```python
from build123d import *

# Parameters (mm, degrees)
SKETCH1_W           = 495.5921
SKETCH1_H           = 147.69846
BOSS_EXTRUDE1_DEPTH = 3.175
SKETCH2_W           = 76.2
SKETCH2_H           = 3.175
BOSS_EXTRUDE2_DEPTH = 6.35
SKETCH3_W           = 3.175
SKETCH3_H           = 188.73216
CUT_EXTRUDE1_DEPTH  = 3.175
SKETCH4_W           = 3.175
SKETCH4_H           = 94.36608
BOSS_EXTRUDE3_DEPTH = 3.175
SKETCH5_W           = 96.57842
SKETCH5_H           = 18.04416
BOSS_EXTRUDE4_DEPTH = 3.175
SKETCH6_W           = 96.577155917
SKETCH6_H           = 2.032
CUT_EXTRUDE2_DEPTH  = 523.024547982
SKETCH7_W           = 6.603370135
SKETCH7_H           = 28.867559882
CUT_EXTRUDE3_DEPTH  = 523.024547982


with BuildPart() as part:
    # Sketch1 → Boss-Extrude1 (new body)
    with BuildSketch(Plane(origin=(0, 0, 0), x_dir=(1, 0, 0), z_dir=(0, 1, 0))):
        with Locations((247.79605, 73.84923)):
            Rectangle(SKETCH1_W, SKETCH1_H)
    extrude(amount=BOSS_EXTRUDE1_DEPTH)

    # Sketch2 → Boss-Extrude2 (add)
    with BuildSketch(Plane(origin=(0, 0, -147.69846), x_dir=(-1, 0, 0), z_dir=(0, 0, -1))):
        with Locations((-447.30289, 1.5875)):
            Rectangle(SKETCH2_W, SKETCH2_H)
        with Locations((-347.54947, 1.5875)):
            Rectangle(SKETCH2_W, SKETCH2_H)
        with Locations((-247.79605, 1.5875)):
            Rectangle(SKETCH2_W, SKETCH2_H)
        with Locations((-148.04263, 1.5875)):
            Rectangle(SKETCH2_W, SKETCH2_H)
        with Locations((-47.895498166, 1.5875)):
            Rectangle(SKETCH2_W, SKETCH2_H)
    extrude(amount=BOSS_EXTRUDE2_DEPTH)

    # Sketch3 → Cut-Extrude1 (cut)
    with BuildSketch(Plane(origin=(0, 3.175, 0), x_dir=(1, 0, 0), z_dir=(0, 1, 0))):
        with Locations((397.42618, 0)):
            Rectangle(SKETCH3_W, SKETCH3_H)
        with Locations((297.67276, 0)):
            Rectangle(SKETCH3_W, SKETCH3_H)
        with Locations((197.91934, 0)):
            Rectangle(SKETCH3_W, SKETCH3_H)
        with Locations((98.167184083, 0)):
            Rectangle(SKETCH3_W, SKETCH3_H)
    extrude(amount=-CUT_EXTRUDE1_DEPTH, mode=Mode.SUBTRACT)

    # Sketch4 → Boss-Extrude3 (add, through all)
    with BuildSketch(Plane(origin=(0, 3.175, 0), x_dir=(1, 0, 0), z_dir=(0, 1, 0))):
        with Locations((-1.5875, 100.51542)):
            Rectangle(SKETCH4_W, SKETCH4_H)
        with Locations((497.1796, 100.51542)):
            Rectangle(SKETCH4_W, SKETCH4_H)
    extrude(amount=-BOSS_EXTRUDE3_DEPTH)

    # Sketch5 → Boss-Extrude4 (add, through all)
    with BuildSketch(Plane(origin=(0, 3.175, 0), x_dir=(1, 0, 0), z_dir=(0, 1, 0))):
        with Locations((247.79605, -9.02208)):
            Rectangle(SKETCH5_W, SKETCH5_H)
        with Locations((347.54947, -9.02208)):
            Rectangle(SKETCH5_W, SKETCH5_H)
        Polygon((429.9839, -18.04416), (431.560448611, -18.04416), (431.560448611, 0), (423.633900075, 0), (399.210535917, 0), (399.210535917, -18.04416), align=None)
        Polygon((495.5921, 0), (484.468648611, -18.04416), (459.500448611, -18.04416), (459.500448611, 0), (484.468648611, 0), align=None)
        Polygon((0, 0), (10.417800633, -18.04416), (96.579684083, -18.04416), (96.579684083, 0), align=None)
    extrude(amount=-BOSS_EXTRUDE4_DEPTH)

    # Sketch6 → Cut-Extrude2 (cut, through all)
    with BuildSketch(Plane(origin=(0, 3.175, 0), x_dir=(1, 0, 0), z_dir=(0, 1, 0))):
        with Locations((148.043262041, 1.016)):
            Rectangle(SKETCH6_W, SKETCH6_H)
    extrude(amount=-CUT_EXTRUDE2_DEPTH, mode=Mode.SUBTRACT)

    # Sketch7 → Cut-Extrude3 (cut, through all)
    with BuildSketch(Plane(origin=(0, 3.175, 0), x_dir=(1, 0, 0), z_dir=(0, 1, 0))):
        with Locations((94.765629101, -7.077939941)):
            Rectangle(SKETCH7_W, SKETCH7_H)
    extrude(amount=-CUT_EXTRUDE3_DEPTH, mode=Mode.SUBTRACT)


solid = part.part
```
The listing builds one solid part. Answer for the finished solid, in the listing's coordinates (mm). Give positions to 0.01 mm unless a question says otherwise; leave off trailing zeros. Order: outer loops, then holes, each group sorted by start corner. A loop starts at its lowest first (then second) coordinate and runs counter-clockwise, first axis right, second up.
Item 1: Find the intervals of material crossed by probe 1 along X at (y, z) = (0.55, -54.5) (3 decimals); probe 2 along X at (y, z) = (1, -53); probe 3 along Z at (x, y) = (102, 0.3), in increasing order.
From the geometry:
probe 1: x = -3.175 to 96.58, 99.755 to 196.332, 199.507 to 296.085, 299.26 to 395.839, 399.014 to 498.767
probe 2: x = 0 to 96.58, 99.75 to 196.33, 199.51 to 296.09, 299.26 to 395.84, 399.01 to 495.59
probe 3: z = -147.7 to -2.03
Item 2: The part is cut by section C-C, the plane x = 452. Give the vertices of the cut face in (y, z) (3 decimals), and give its area (3 significant figures).
From the geometry:
outline: (0, -154.048) - (3.175, -154.048) - (3.175, 0) - (0, 0) - close
area: 489 mm2
Item 3: The part is cut by section A-A, the plane z = -23. Give the vertices of the cut face in (x, y) (3 decimals).
From the geometry:
outline: (0, 0) - (96.58, 0) - (96.58, 3.175) - (0, 3.175) - close; (99.755, 0) - (196.332, 0) - (196.332, 3.175) - (99.755, 3.175) - close; (199.507, 0) - (296.085, 0) - (296.085, 3.175) - (199.507, 3.175) - close; (299.26, 0) - (395.839, 0) - (395.839, 3.175) - (299.26, 3.175) - close; (399.014, 0) - (495.592, 0) - (495.592, 3.175) - (399.014, 3.175) - close
Item 4: Given pin 1 Ø1 at (y, z) = (1, 10) entering from -X; pin 2 Ø1 at (x, y) = (102, 2) entering from -Z; pin 3 Ø1 at (y, z) = (1.5, -10) entering from +X, each flat-ended and moving along its own axis, determine where each tip first touches the part or whether it passes through.
From the geometry:
pin 1: stops at x = 5.48
pin 2: stops at z = -147.7
pin 3: stops at x = 495.59
Item 5: The part is cut by section B-B, the plane x = 179. Give the vertices of the cut face in (y, z) (3 decimals).
From the geometry:
outline: (0, -154.048) - (3.175, -154.048) - (3.175, -2.032) - (0, -2.032) - close
